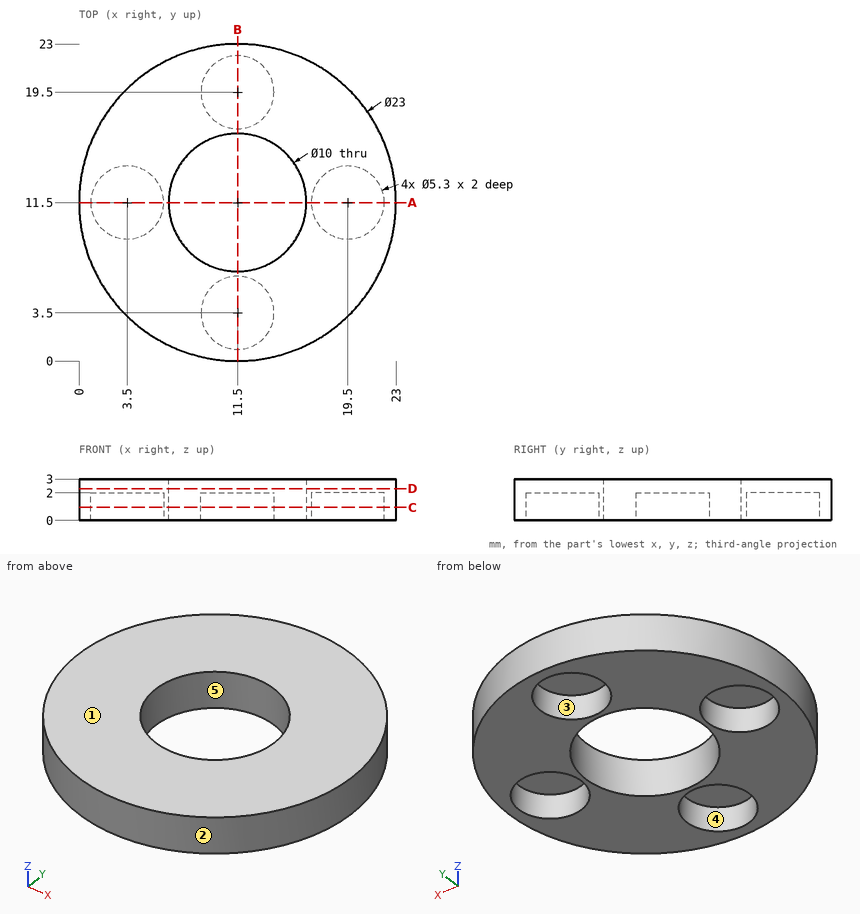
Here's the drawing with two shaded views (mm, measured from the low corner). I have some questions. A direction names the side the tool comes from. Coordinates: 2 decimals unless noted, no trailing zeros. Loops run counter-clockwise (first coordinate to the right, second up) from the corner with the lowest first, then second, coordinate; pieces in that order, holes last. Notation, with made-up numbers: (22.25, 53.5) -> (35.25, 53.5) arc R11 cw to (35.25, 63.5) -> close; hole circle Ø8 at (-0.5, -7). An arc over 180 degrees is marked (long way). Use one line per item in the form item = value. Start each with the question number.
(1) If we section it at A-A (y = 11.5): Please give me the cut outline in (x, z), then the cut area to 3 significant figures.
(2) Please list where these lines run through material, in increasing order: line 1 along Y through (x, z) = (11.5, 1.15); line 2 along Y through (x, z) = (11.5, 2.45); line 3 along X through (y, z) = (11.75, 1.4).
(3) Will these pins go through, and if not, where does the flat tip stop? pin 1 (1.6 mm diameter, centred on x = 20.5, y = 10.5, fed in from -Z); pin 2 (1.5 mm diameter, centred on y = 16, z = 1, fed in from -X).
(4) We'd pull the mould along Y, two halves only. Please class the marked faces 1, 2 and 3: pulls with the +Y half, pulls with the -Y half, needs draft (parallel to the pull), parting line crosses it, or undercut.
(5) If we section it at D-D (z = 2.3): Please give me the cut outline in (x, y).
(6) If we section it at C-C (z = 0.95): Please give me the cut outline in (x, y), then the cut area to 3 significant figures.
(7) On a 3-axis mill with a long thin cutter (end or side, diameter ignored), from which of +Z, -Z, +X, -X, +Y, -Y can I reach the whole of each face in a straight line? I mean the marked faces 4 and 5. Say none if no direction works.
Verdict:
q1.outline = (0, 0) -> (0.85, 0) -> (0.85, 2) -> (6.15, 2) -> (6.15, 0) -> (6.5, 0) -> (6.5, 3) -> (0, 3) -> close; (16.5, 0) -> (16.85, 0) -> (16.85, 2) -> (22.15, 2) -> (22.15, 0) -> (23, 0) -> (23, 3) -> (16.5, 3) -> close
q1.area = 17.8 mm²
q2.line_1 = 0 to 0.85, 6.15 to 6.5, 16.5 to 16.85, 22.15 to 23
q2.line_2 = 0 to 6.5, 16.5 to 23
q2.line_3 = 0 to 0.86, 6.14 to 6.51, 16.49 to 16.86, 22.14 to 23
q3.pin_1 = 2
q3.pin_2 = 0.63
q4.face_1 = needs draft
q4.face_2 = parting line crosses it
q4.face_3 = undercut
q5.outline = circle Ø23 at (11.5, 11.5); hole circle Ø10 at (11.5, 11.5)
q6.outline = circle Ø23 at (11.5, 11.5); hole circle Ø5.3 at (3.5, 11.5); hole circle Ø10 at (11.5, 11.5); hole circle Ø5.3 at (11.5, 3.5); hole circle Ø5.3 at (11.5, 19.5); hole circle Ø5.3 at (19.5, 11.5)
q6.area = 249 mm²
q7.face_4 = -Z
q7.face_5 = +Z, -Z
